For this review, take the finished solid that the model builds, in its own axes (mm). A direction names the side the tool comes from. Give positions to 0.01 mm unless a question says otherwise; leave off trailing zeros. Write each loop counter-clockwise with the first axis right and the second up, starting at its lowest first coordinate (ties: lowest second). Pieces come first, ordered by that corner, then holes. Notation, with made-up numbers: M 13.25,4.5 L 66.25,4.5 A32 cw 66.25,41.5 Z; hole C 47.25,-14.5 d3. An arc over 180 degrees is marked long. Answer as a JSON object with one key per item and string values. Group by question number.
```python
from build123d import *

# Parameters (mm, degrees)
SKETCH_1_W          = 40.2
SKETCH_1_H          = 70
EXTRUDE_1_DEPTH     = 2
SKETCH_2_W          = 2
SKETCH_2_H          = 6.1
SKETCH_2_H_2        = 6.45
CUT_EXTRUDE_1_DEPTH = 81.746764641
SKETCH_3_W          = 6
SKETCH_3_H          = 2
EXTRUDE_2_DEPTH     = 2
SKETCH_4_W          = 5
SKETCH_4_H          = 2
EXTRUDE_3_DEPTH     = 5
CUT_EXTRUDE_2_DEPTH = 86.117800723
CUT_EXTRUDE_3_DEPTH = 5
SKETCH_8_W          = 2
SKETCH_8_H          = 2
CUT_EXTRUDE_4_DEPTH = 5


with BuildPart() as part:
    # ｽｹｯﾁ1 → ﾎﾞｽ - 押し出し1 (new body)
    with BuildSketch(Plane(origin=(0, 0, 0), x_dir=(1, 0, 0), z_dir=(0, 1, 0))):
        with Locations((20.1, 35)):
            Rectangle(SKETCH_1_W, SKETCH_1_H)
    extrude(amount=EXTRUDE_1_DEPTH)

    # ｽｹｯﾁ2 → ｶｯﾄ - 押し出し1 (cut, through all)
    with BuildSketch(Plane(origin=(0, 2, 0), x_dir=(1, 0, 0), z_dir=(0, 1, 0))):
        with Locations((1, 13.3)):
            Rectangle(SKETCH_2_W, SKETCH_2_H)
        with Locations((39.2, 13.3)):
            Rectangle(SKETCH_2_W, SKETCH_2_H)
        with Locations((1, 61.775)):
            Rectangle(SKETCH_2_W, SKETCH_2_H_2)
        with Locations((39.2, 61.775)):
            Rectangle(SKETCH_2_W, SKETCH_2_H_2)
    extrude(amount=-CUT_EXTRUDE_1_DEPTH, mode=Mode.SUBTRACT)

    # ｽｹｯﾁ3 → ﾎﾞｽ - 押し出し2 (add)
    with BuildSketch(Plane.XY):
        with Locations((5, 1)):
            Rectangle(SKETCH_3_W, SKETCH_3_H)
        with Locations((35.2, 1)):
            Rectangle(SKETCH_3_W, SKETCH_3_H)
    extrude(amount=EXTRUDE_2_DEPTH)

    # ｽｹｯﾁ4 → ﾎﾞｽ - 押し出し3 (add)
    with BuildSketch(Plane(origin=(0, 0, -70), x_dir=(-1, 0, 0), z_dir=(0, 0, -1))):
        with Locations((-35.7, 1)):
            Rectangle(SKETCH_4_W, SKETCH_4_H)
        with Locations((-4.5, 1)):
            Rectangle(SKETCH_4_W, SKETCH_4_H)
    extrude(amount=EXTRUDE_3_DEPTH)

    # ｽｹｯﾁ5 → ｶｯﾄ - 押し出し2 (cut, through all)
    with BuildSketch(Plane(origin=(0, 2, 0), x_dir=(1, 0, 0), z_dir=(0, 1, 0))):
        Polygon((7, 75), (2, 70), (2, 75), align=None)
        Polygon((33.2, 75), (38.2, 70), (38.2, 75), align=None)
    extrude(amount=-CUT_EXTRUDE_2_DEPTH, mode=Mode.SUBTRACT)

    # ｽｹｯﾁ7 → ｶｯﾄ - 押し出し3 (cut)
    with BuildSketch(Plane(origin=(0, 2, 0), x_dir=(1, 0, 0), z_dir=(0, 1, 0))):
        Polygon((14.1, 70), (14.1, 47), (20.1, 43.5), (26.1, 47), (26.1, 70), align=None)
    extrude(amount=-CUT_EXTRUDE_3_DEPTH, mode=Mode.SUBTRACT)

    # ｽｹｯﾁ8 → ｶｯﾄ - 押し出し4 (cut)
    with BuildSketch(Plane(origin=(0, 2, 0), x_dir=(1, 0, 0), z_dir=(0, 1, 0))):
        with Locations((12.025, 62.71)):
            Rectangle(SKETCH_8_W, SKETCH_8_H)
        with Locations((12.025, 52.91)):
            Rectangle(SKETCH_8_W, SKETCH_8_H)
        with Locations((28.175, 62.71)):
            Rectangle(SKETCH_8_W, SKETCH_8_H)
        with Locations((28.175, 52.91)):
            Rectangle(SKETCH_8_W, SKETCH_8_H)
    extrude(amount=-CUT_EXTRUDE_4_DEPTH, mode=Mode.SUBTRACT)


solid = part.part
```
Item 1: Consider section A-A (z = -50). Give the boundary of the cut face in (x, y).
Item 2: Consider section C-C (x = 31.5). Give the boundary of the cut face in (y, z).
Item 3: Insertion check: P1, Ø1, axis at x = 39.5, y = 0.5, coming from the +Z side; P2, Ø1, axis at y = 1.5, z = 1, coming from the +X side; P3, Ø0.6, axis at x = 11.5, y = 1, coming from the -Z side; P4, Ø6, axis at x = 19, z = -57.5, coming from the +Y side. Each pin has a flat end and moves straight along its axis. Give the tip position at first contact, or say it passes through.
Item 4: Draft analysis for pull direction Z (two halves, no side actions). For faces 5 (the flat face through (0, 1, -5)), 6 (the flat face through (12, 1, -53.91)), 7 (the flat face through (1, 1, 0)), state which applies: released by +Z, released by -Z, zero draft, split by the parting line, or undercut.
Item 5: To check wall thickness, follow probe 1 along Z at (x, y) = (12, 0.55); probe 2 along X at (y, z) = (1.4, -69); probe 3 along X at (y, z) = (0.75, -60.5). State the ranges of each line that lie inside material, in increasing order.
Item 6: Consider section B-B (y = 1.55). State how many separate pieces and enclosed holes the cut face has, plus the area to 3 significant figures.
Item 7: Machinability: for faces 1 (the flat face through (30, 1, -70)), 2 (the flat face through (39, 1, -58.55)), 3 (the flat face through (11.025, 1, -63)), 4 (the flat face through (1, 1, -10.25)), which of the approach directions +Z, -Z, +X, -X, +Y, -Y give a long, thin tool a straight path to every point of the face, cutting with its end or side? Answer none if there is none.
Item 8: Consider section D-D (x = 37). Give the boundary of the cut face in (y, z), plus the area to 3 significant figures.
Result set:
{
 "1": {"outline": "M 0,0 L 14.1,0 L 14.1,2 L 0,2 Z; M 26.1,0 L 40.2,0 L 40.2,2 L 26.1,2 Z"},
 "2": {"outline": "M 0,-70 L 2,-70 L 2,0 L 0,0 Z"},
 "3": {"P1": "stops at z = 0", "P2": "stops at x = 38.2", "P3": "stops at z = -70", "P4": "passes through"},
 "4": {"face 5": "zero draft", "face 6": "undercut", "face 7": "released by +Z"},
 "5": {"probe 1": "z = -70 to -63.71, -61.71 to -53.91, -51.91 to 0", "probe 2": "x = 0 to 14.1, 26.1 to 40.2", "probe 3": "x = 2 to 14.1, 26.1 to 38.2"},
 "6": {"separate pieces": "1", "enclosed holes": "4", "area": "2,500 mm^2"},
 "7": {"face 1": "-Z, +Y, -Y", "face 2": "+X, +Y, -Y", "face 3": "+Y, -Y", "face 4": "-X, +Y, -Y"},
 "8": {"outline": "M 0,-71.2 L 2,-71.2 L 2,2 L 0,2 Z", "area": "146 mm^2"}
}
